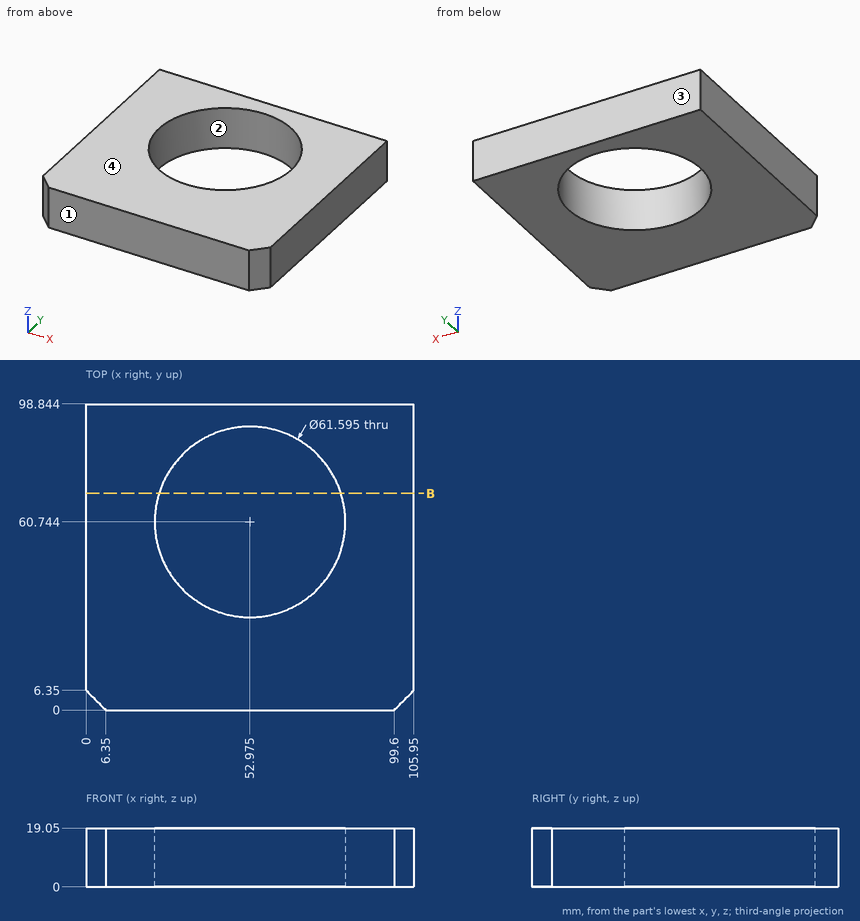
Answer from the drawing. Dimensions are ordinates in mm from the lowest x, y and z of the part. Coordinates: 2 decimals unless noted, no trailing zeros. Order: outer loops, then holes, each group sorted by start corner. A loop starts at its lowest first (then second) coordinate and runs counter-clockwise, first axis right, second up. Notation, with made-up numbers: (-17.5, 6) - (15.5, 6) arc R18 cw to (15.5, 36) - close; hole circle Ø6 at (-0.5, 83.25). An arc over 180 degrees is marked (long way). Answer as a JSON object with one key per item and string values. Group by question number.
Item 1: A flat-ended cylindrical pin translates along its axis: P1, Ø5, axis at x = 24, y = 69, coming from the +Z side. Find the tip coordinate at first contact, or state that the pin passes through.
Item 2: Consider probe 1 along X at (y, z) = (39.5, 14.5); probe 2 along X at (y, z) = (42.5, 9.5); probe 3 along Y at (x, z) = (36, 13.5) (1 decimal). Determine where each line is inside the solid, lowest interval first. Write a range as from..to.
Item 3: The mould has two halves that part along Y. Classify the marked faces 1, 2, 3 and 4: +Y half, -Y half, draft (parallel to the pull), parting line (faces both ways), or undercut.
Item 4: Section B-B (y = 70) is taken. Give the vertices of the cut face in (x, z).
Results are:
{
 "1": {"P1": "stops at z = 19.05"},
 "2": {"probe 1": "x = 0..30.68, 75.27..105.95", "probe 2": "x = 0..28.16, 77.79..105.95", "probe 3": "y = 0..35, 86.4..98.8"},
 "3": {"face 1": "-Y half", "face 2": "undercut", "face 3": "+Y half", "face 4": "draft"},
 "4": {"outline": "(0, 0) - (23.6, 0) - (23.6, 19.05) - (0, 19.05) - close; (82.35, 0) - (105.95, 0) - (105.95, 19.05) - (82.35, 19.05) - close"}
}
